CAD build for the part. Positions are in the model's coordinates, mm. Round coordinates to 2 decimals unless told otherwise and drop trailing zeros. Loops run counter-clockwise (first coordinate to the right, second up) from the corner with the lowest first, then second, coordinate; pieces in that order, holes last. Notation, with made-up numbers: (-4.5, -12) -> (49.5, -12) arc R27 ccw to (49.5, 21) -> close; hole circle Ø5 at (62, 6). An arc over 180 degrees is marked (long way). Answer as CSV lines item,"result".
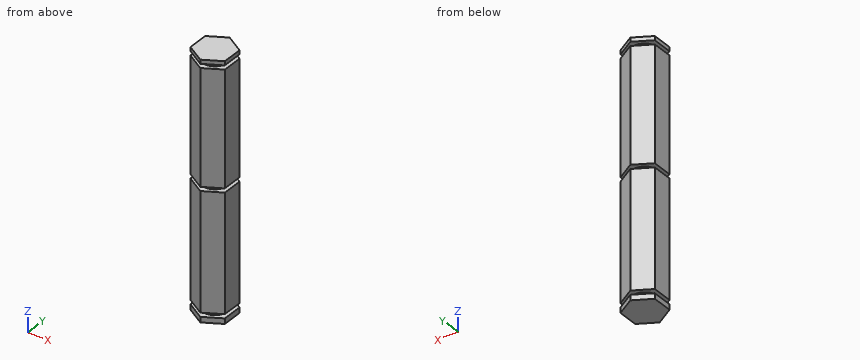
Autodesk Inventor part; units mm, degrees
ref_plane "YZ Plane" through (0, 0, 0) normal (1, 0, 0) x (0, 1, 0)
ref_plane "XZ Plane" through (0, 0, 0) normal (0, 1, 0) x (-1, 0, 0)
ref_plane "XY Plane" through (0, 0, 0) normal (0, 0, 1) x (1, 0, 0)
sketch "Sketch1" plane through (0, 0, 0) normal (0, 0, 1) x (1, 0, 0)
  line L0 (6.35, -3.6662) -> (0, -7.3323)
  line L1 (0, -7.3323) -> (-6.35, -3.6662)
  line L2 (-6.35, -3.6662) -> (-6.35, 3.6662)
  line L3 (-6.35, 3.6662) -> (0, 7.3323)
  line L4 (0, 7.3323) -> (6.35, 3.6662)
  line L5 (6.35, 3.6662) -> (6.35, -3.6662)
  point P0 (0, 0)
  point P1 (0, 0)
  dimension "d0" = 12.7
extrude "Extrusion1" add sketch "Sketch1" along normal blind 94
sketch "Sketch2" plane through (0, 0, 0) normal (1, 0, 0) x (0, 1, 0)
  line L0 (15, 2) -> (5, 2)
  line L1 (5, 2) -> (5, 3.5)
  line L2 (5, 3.5) -> (15, 3.5)
  line L3 (15, 3.5) -> (15, 2)
  line L4 (3.6662, 0) -> (7.3323, 0)
  line L5 (0, -18.42) -> (0, 110.52)
  line L6 (15, 92.5) -> (5, 92.5)
  line L7 (5, 92.5) -> (5, 91)
  line L8 (5, 91) -> (15, 91)
  line L9 (15, 91) -> (15, 92.5)
  line L10 (15, 48.5) -> (5, 48.5)
  line L11 (5, 48.5) -> (5, 47)
  line L12 (5, 47) -> (15, 47)
  line L13 (15, 47) -> (15, 48.5)
  point P0 (0, 0)
  point P1 (0, 0)
  point P2 (15, 2.75)
  point P3 (15, 47.75)
  dimension "d3" = 1.5
  dimension "d4" = 2
  dimension "d5" = 10
  dimension "d6" = 5
  dimension "d8" = 91
  dimension "d9" = 47
revolve "Revolution1" cut sketch "Sketch2" angle 360 about axis through (0, 0, -10) along (0, 0, 1)
properties part number "Drive Shaft"
Q1. Drop flat-ended pins along their axis: pin 1 Ø3 at (x, z) = (0, 11.5) entering from +Y; pin 2 Ø1 at (x, z) = (-2.5, 27) entering from -Y. Give the stop position or say it passes through.
Results:
pin 1,"y = 7.33"
pin 2,"y = -6.18"
Q2. Slice it at A-A, the plane y = 6. Give the cut face in (x, z), and give its area (3 significant figures).
Results:
outline,"(-2.31, 0) -> (2.31, 0) -> (2.31, 2) -> (-2.31, 2) -> close; (-2.31, 3.5) -> (2.31, 3.5) -> (2.31, 47) -> (-2.31, 47) -> close; (-2.31, 48.5) -> (2.31, 48.5) -> (2.31, 91) -> (-2.31, 91) -> close; (-2.31, 92.5) -> (2.31, 92.5) -> (2.31, 94) -> (-2.31, 94) -> close"
area,"413 mm2"
Q3. Probe L1, parallel to Z at x = 5.75, y = 1.75; L2, parallel to Y at x = -5.5, z = 83; L3, parallel to Y at x = -1.25, z = 87. List the from-to ranges inside material, lowest first. Write a range as [from, to].
Results:
L1,"[0, 2], [3.5, 47], [48.5, 91], [92.5, 94]"
L2,"[-4.16, 4.16]"
L3,"[-6.61, 6.61]"
Q4. Slice it at C-C, the plane z = 25. Give the cut face in (x, y), and give its area (3 significant figures).
Results:
outline,"(-6.35, -3.67) -> (0, -7.33) -> (6.35, -3.67) -> (6.35, 3.67) -> (0, 7.33) -> (-6.35, 3.67) -> close"
area,"140 mm2"
Q5. Slice it at B-B, the plane x = 1. Give the cut face in (y, z), and give its area (3 significant figures).
Results:
outline,"(-6.75, 0) -> (6.75, 0) -> (6.75, 2) -> (4.9, 2) -> (4.9, 3.5) -> (6.75, 3.5) -> (6.75, 47) -> (4.9, 47) -> (4.9, 48.5) -> (6.75, 48.5) -> (6.75, 91) -> (4.9, 91) -> (4.9, 92.5) -> (6.75, 92.5) -> (6.75, 94) -> (-6.75, 94) -> (-6.75, 92.5) -> (-4.9, 92.5) -> (-4.9, 91) -> (-6.75, 91) -> (-6.75, 48.5) -> (-4.9, 48.5) -> (-4.9, 47) -> (-6.75, 47) -> (-6.75, 3.5) -> (-4.9, 3.5) -> (-4.9, 2) -> (-6.75, 2) -> close"
area,"1,250 mm2"
